Work out the finished part from the listing and answer in its coordinate system (mm). Coordinates: 2 decimals unless noted, no trailing zeros. Order: outer loops, then holes, each group sorted by start corner. A loop starts at its lowest first (then second) coordinate and runs counter-clockwise, first axis right, second up. Notation, with made-up numbers: (-30.5, 7) -> (-8.5, 7) arc R21 ccw to (-8.5, 43) -> close; hole circle Ø2 at (-13, 35). An arc over 180 degrees is marked (long way). Use one line per item in the form item = value.
from build123d import *

# Parameters (mm, degrees)
F0_W     = 2000
F0_H     = 1000
F1_DEPTH = 25
F2_W     = 100
F2_H     = 100
F4_DEPTH = 700
F3_R     = 25
F3_R_2   = 26.6431742527
F5_DEPTH = 1000.001
F6_R     = 138.4561690077
F7_W     = 118.5409426689
F7_H     = 157.5430333614
F9_T     = 2.5


# Not quite as in the source:
# - a pattern or mirror of a feature is missing from the dataset's text; its kind, count and spacing are read off the source's solid
# - a shell that OpenCascade refuses in one call is made with other operations: the cavity is built on its own and cut out


with BuildPart() as f1:
    # F0 (on Top) → F1 (new body)
    with BuildSketch(Plane.XY):
        Rectangle(F0_W, F0_H)
    extrude(amount=F1_DEPTH)

    # F2 (on face) → F4 (join)
    with BuildSketch(Plane(origin=(0, 0, 0), x_dir=(1, 0, 0), z_dir=(0, 0, -1))):
        with Locations((-950, 450)):
            Rectangle(F2_W, F2_H)
        with Locations((-950, -450)):
            Rectangle(F2_W, F2_H)
    f4 = extrude(amount=F4_DEPTH)

    # F4_copies: F4 across plane
    add(f4.mirror(Plane(origin=(0, 0, 0), x_dir=(0, 0, 1), z_dir=(1, 0, 0))))

    # F3 (on face) → F5 (cut, through all)
    with BuildSketch(Plane.XZ.offset(500)):
        with Locations((-950, -100)):
            Circle(F3_R)
        with Locations((-950, -300)):
            Circle(F3_R)
        with Locations((-950, -500)):
            Circle(F3_R_2)
    f5 = extrude(amount=-F5_DEPTH, mode=Mode.SUBTRACT)

    # F5_copies: F5 across plane
    add(f5.mirror(Plane(origin=(0, 0, 0), x_dir=(0, 0, 1), z_dir=(1, 0, 0))), mode=Mode.SUBTRACT)


with BuildPart() as f8:
    # F6 (on face) → F8 section 0
    with BuildSketch(Plane.XZ.offset(500)):
        with Locations((508.7250471115, -680.1778674126)):
            Circle(F6_R)
    # F7 (on face) → F8 section 1
    with BuildSketch(Plane.YZ.offset(-900)):
        with Locations((720.3351557255, -315.4024332762)):
            Rectangle(F7_W, F7_H)
    loft()

    # F9: shell of thickness 2.5, made by hand


with BuildPart() as f9_core1:
    # F9_t2: copy of F8
    add(f8.part)

    # the walls: a layer under each face that stays
    f9_faces = [f9_core1.faces().sort_by_distance(p)[0] for p in [
        (508.7250471115, -500, -680.1778674126),
        (-900, 720.3351557255, -315.4024332762),
    ]]
    thicken(f9_faces, amount=-F9_T, mode=Mode.SUBTRACT)


with BuildPart() as f8_1:
    add(f8.part)

    # what is left inside the walls is the cavity
    f9_cavity = [f9_core1.part.solids().sort_by_distance(p)[0] for p in [
        (-53.137215, -112.959985, -558.586056),
    ]]
    add(f9_cavity, mode=Mode.SUBTRACT)


solid = f1.part
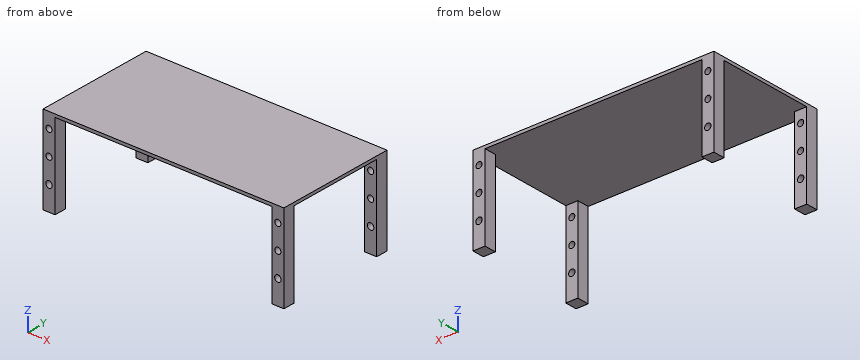
(1) Section A-A on z = -500 is taken. Count the separate pieces of the cut face and the enclosed holes in it, plus the area to 3 significant figures.
Data:
separate_pieces = 8
enclosed_holes = 0
area = 18,700 mm²
(2) Section C-C on z = -371.5 is taken. Write down the section's boundary in (x, y), plus the area to 3 significant figures.
Data:
outline = (-1000, -500) -> (-900, -500) -> (-900, -400) -> (-1000, -400) -> close; (-1000, 400) -> (-900, 400) -> (-900, 500) -> (-1000, 500) -> close; (900, -500) -> (1000, -500) -> (1000, -400) -> (900, -400) -> close; (900, 400) -> (1000, 400) -> (1000, 500) -> (900, 500) -> close
area = 40,000 mm²
(3) Straight lines are drawn through the part: line 1 along Z through (x, y) = (950, -428.5); line 2 along X through (y, z) = (-415, -21); line 3 along Z through (x, y) = (-311, -25.5). For each, find the intervals that lie inside material, in ascending order.
Data:
line_1 = -700 to -526.64, -473.36 to -325, -275 to -125, -75 to 25
line_2 = -1000 to -900, 900 to 1000
line_3 = 0 to 25
(4) Section D-D on y = -97.5 is taken. Write down the section's boundary in (x, z), plus the area to 3 significant figures.
Data:
outline = (-1000, 0) -> (1000, 0) -> (1000, 25) -> (-1000, 25) -> close
area = 50,000 mm²
(5) Each of these flat-tipped pins is pushed along its axis until it touches: P1, Ø12, axis at y = -393, z = -259, coming from the +X side; P2, Ø1.5, axis at x = 307.5, y = 292, coming from the -Z side. Where does it stop, or does it pass through?
Data:
P1 = through
P2 = 0
